Can you work these out from the model? Positions are in its coordinate system, mm. Coordinates: 2 decimals unless noted, no trailing zeros. Loops run counter-clockwise (first coordinate to the right, second up) from the corner with the lowest first, then second, coordinate; pieces in that order, holes last. Notation, with made-up numbers: M 30,59 L 74,59 A23 ccw 74,78 Z; hole C -3,-36.75 d4. An arc over 180 degrees is marked long. Return JSON: item names as keys, results as strings. Group by question number.
```python
from build123d import *

# Parameters (mm, degrees)
F0_W          = 900
F0_H          = 50
F1_DEPTH      = 18
F2_R          = 3
F3_DEPTH      = 25
F4_DEPTH      = 900.001
F4_DEPTH_BACK = 25


with BuildPart() as f1:
    # F0 (on Front) → F1 (new body)
    with BuildSketch(Plane.XZ):
        with Locations((450, 25)):
            Rectangle(F0_W, F0_H)
    extrude(amount=F1_DEPTH)

    # F2 (on face) → F3 (cut)
    with BuildSketch(Plane(origin=(0, 0, 0), x_dir=(0, -1, 0), z_dir=(-1, 0, 0))):
        with Locations((9, 25)):
            Circle(F2_R)
    extrude(amount=-F3_DEPTH, mode=Mode.SUBTRACT)

    # F2 (on face) → F4 (cut, two sides)
    with BuildSketch(Plane(origin=(0, 0, 0), x_dir=(0, -1, 0), z_dir=(-1, 0, 0))) as f4_sk:
        with Locations((9, 25)):
            Circle(F2_R)
    extrude(amount=-F4_DEPTH, mode=Mode.SUBTRACT)
    extrude(f4_sk.sketch, amount=-F4_DEPTH_BACK, mode=Mode.SUBTRACT)


solid = f1.part
```
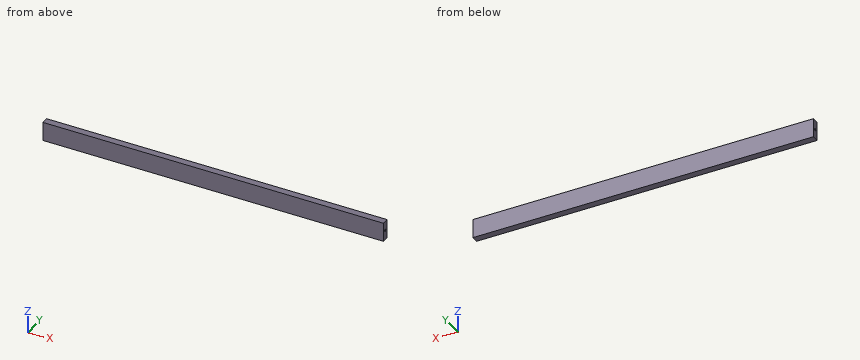
1) Suppose I cut it at A-A, the plane y = -9. List the corners of the cut face in (x, z) for me, then the cut area to 3 significant figures.
2) If I drill on line 1 (Z direction, x = 675, y = -9); line 2 (Z direction, x = 330.5, y = -6.75); line 3 (Y direction, x = 698.5, z = 22.5), over which ranges is the centre line in solid material (lowest first)? Write a range as from..to.
3) Suppose I cut it at B-B, the plane x = 129. List the corners of the cut face in (y, z) for me.
Returned:
{
 "1": {"outline": "M 0,0 L 900,0 L 900,22 L 0,22 Z; M 0,28 L 900,28 L 900,50 L 0,50 Z", "area": "39,600 mm²"},
 "2": {"line 1": "z = 0..22, 28..50", "line 2": "z = 0..23.02, 26.98..50", "line 3": "y = -18..-10.66, -7.34..0"},
 "3": {"outline": "M -18,0 L 0,0 L 0,50 L -18,50 Z; hole C -9,25 d6"}
}
